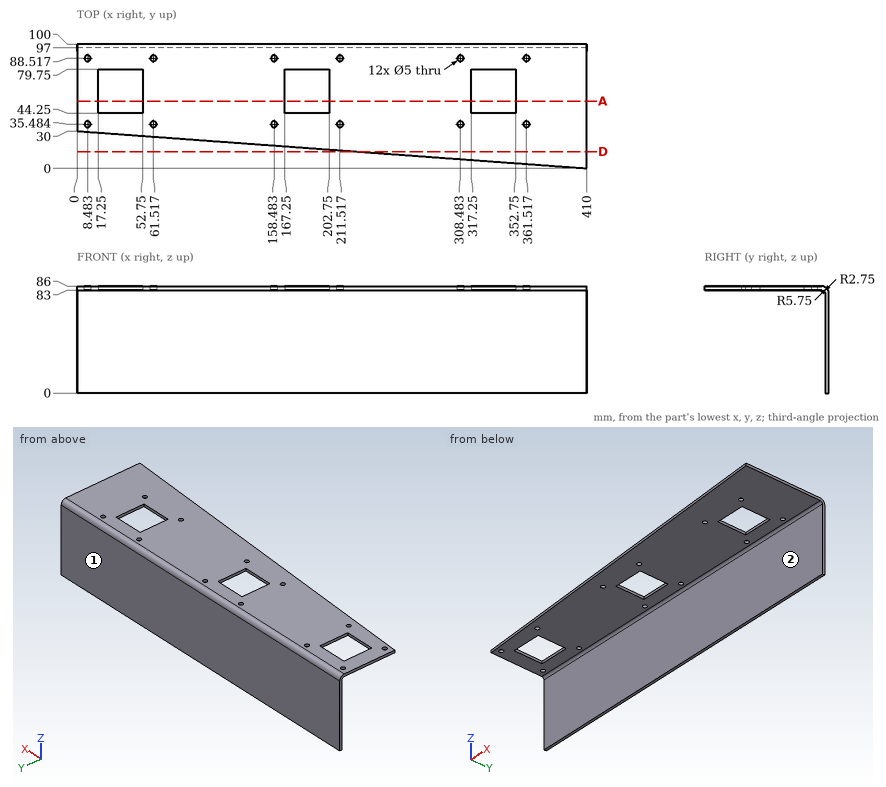
Study the drawing (mm; zero at the part's minimum x, y, z) and answer. A direction names the side the tool comes from. Coordinates: 2 decimals unless noted, no trailing zeros. Write each loop counter-clockwise with the first axis right and the second up, starting at its lowest first coordinate (ties: lowest second). Pieces come first, ordered by that corner, then holes. Notation, with made-up numbers: (62.5, 7) - (73.5, 7) arc R18 cw to (73.5, 27) - close; hole circle Ø3 at (-28.75, -22.75). An arc over 180 degrees is marked (long way). Answer as a JSON object with one key per item and string values.
Q1. Which of the six approach directions +Z, -Z, +X, -X, +Y, -Y give full straight-line access (tool end or side, diameter ignored) to the marked faces 1 and 2?
Results list:
{"face 1": "+Z, -Z, +X, -X, +Y", "face 2": "-Z, +X, -X, -Y"}
Q2. Consider L1, parallel to Y at x = 198, z = 47; L2, parallel to Z at x = 19.5, y = 39. Determine where each line is inside the solid, lowest interval first. Write a range as from..to.
Results list:
{"L1": "y = 97..100", "L2": "z = 83..86"}
Q3. Find section A-A (y = 54). Write down the section's boundary in (x, z).
Results list:
{"outline": "(0, 83) - (17.25, 83) - (17.25, 86) - (0, 86) - close; (52.75, 83) - (167.25, 83) - (167.25, 86) - (52.75, 86) - close; (202.75, 83) - (317.25, 83) - (317.25, 86) - (202.75, 86) - close; (352.75, 83) - (410, 83) - (410, 86) - (352.75, 86) - close"}
Q4. Given pin 1 Ø6.5 at (x, y) = (308.48, 88.52) entering from -Z; pin 2 Ø2.5 at (x, z) = (183.5, 84.5) entering from +Y (1 decimal); pin 3 Ø0.9 at (x, z) = (182.5, 84.5) entering from -Y, each flat-ended and moving along its own axis, determine where each tip first touches the part or whether it passes through.
Results list:
{"pin 1": "stops at z = 83", "pin 2": "stops at y = 99.2", "pin 3": "stops at y = 16.61"}
Q5. Find section D-D (y = 13.5). Write down the section's boundary in (x, z).
Results list:
{"outline": "(225.5, 83) - (410, 83) - (410, 86) - (225.5, 86) - close"}
